```python
from build123d import *

# Parameters (mm, degrees)
SKETCH1_R           = 3.302
BOSS_EXTRUDE1_DEPTH = 19.05
CHAMFER1_SIZE       = 6.593417442
CHAMFER1_SIZE_2     = 6.35
FILLET1_R           = 5.08
FILLET2_R           = 1.27
FILLET3_R           = 1.27
BOSS_EXTRUDE2_START = 38.1
BOSS_EXTRUDE2_DEPTH = 38.1
FILLET5_R           = 2.54
FILLET6_R           = 1.27
SKETCH7_W           = 12.7
SKETCH7_H           = 19.05
BOSS_EXTRUDE3_DEPTH = 12.7
CUT_EXTRUDE5_REACH  = 244.877
SKETCH8_R           = 3.302
SKETCH9_W           = 12.7
SKETCH9_H           = 19.05
BOSS_EXTRUDE4_DEPTH = 12.7
CUT_EXTRUDE6_REACH  = 261.3
SKETCH10_R          = 3.302
FILLET7_R           = 1.27


with BuildPart() as part:
    # Sketch1 → Boss-Extrude1 (new body)
    with BuildSketch(Plane(origin=(0, 0, 0), x_dir=(1, 0, 0), z_dir=(0, 1, 0))):
        with BuildLine():
            Line((0, 0), (0, -107.95))
            ThreePointArc((0, -107.95), (44.047088178, -127.137896363), (63.234984541, -171.184984541))
            Line((63.234984541, -171.184984541), (171.184984541, -171.184984541))
            Line((171.184984541, -171.184984541), (171.184984541, -172.327984541))
            Line((171.184984541, -172.327984541), (173.724984541, -172.327984541))
            Line((173.724984541, -172.327984541), (171.184984541, -168.644984541))
            Line((171.184984541, -168.644984541), (171.184984541, -139.434984541))
            Line((171.184984541, -139.434984541), (158.484984541, -139.434984541))
            Line((158.484984541, -139.434984541), (158.484984541, -152.134984541))
            Line((158.484984541, -152.134984541), (78.172986392, -152.134984541))
            ThreePointArc((78.172986392, -152.134984541), (56.455029962, -114.729954579), (19.05, -93.011998149))
            Line((19.05, -93.011998149), (19.05, -12.7))
            Line((19.05, -12.7), (31.75, -12.7))
            Line((31.75, -12.7), (31.75, 0))
            Line((31.75, 0), (2.54, 0))
            Line((2.54, 0), (-1.143, 2.54))
            Line((-1.143, 2.54), (-1.143, 0))
            Line((-1.143, 0), (0, 0))
        make_face()
        with Locations(Location((25.4, -6.35, 0), (0, 0, 90))):
            Circle(SKETCH1_R, mode=Mode.SUBTRACT)
        with Locations(Location((164.834984541, -145.784984541, 0), (0, 0, 90))):
            Circle(SKETCH1_R, mode=Mode.SUBTRACT)
    extrude(amount=BOSS_EXTRUDE1_DEPTH)

    # Chamfer1
    # the kernel refuses this chamfer: 6.593417442, 6.35 mm, written as the material it takes off along each edge
    with BuildSketch(Plane(origin=(63.234984541, -17.246656522, 171.184984541), x_dir=(-0.0872058515963271, 0, -0.9961903128656489), z_dir=(0, 1, 0))) as chamfer1_piece_1:
        with BuildLine():
            Line((6.700635555, 0), (-CHAMFER1_SIZE * 0.0872058515927, -CHAMFER1_SIZE * 0.996190312824))
            Line((-CHAMFER1_SIZE * 0.0872058515927, -CHAMFER1_SIZE * 0.996190312824), (0, 0))
            ThreePointArc((0, 0), (3.448459053, -0.085459063), (6.700635555, 0))
        make_face()
    extrude(amount=53.543313044, mode=Mode.SUBTRACT)
    with BuildSketch(Plane(origin=(0, -18.02411909, 107.95), x_dir=(0, 0, -1), z_dir=(0, 1, 0))) as chamfer1_piece_2:
        with BuildLine():
            Line((CHAMFER1_SIZE_2, 0), (-0.627104296, -6.977104296))
            ThreePointArc((-0.627104296, -6.977104296), (-0.229600221, -3.597999822), (0, 0))
            Line((0, 0), (CHAMFER1_SIZE_2, 0))
        make_face()
    extrude(amount=55.098238181, mode=Mode.SUBTRACT)

    # Fillet1
    fillet1_edges = [part.edges().sort_by_distance(p)[0] for p in [
        (19.05, 9.525, 93.011998149),
        (78.172986392, 9.525, 152.134984541),
    ]]
    fillet(fillet1_edges, radius=FILLET1_R)

    # Fillet2
    fillet2_edges = [part.edges().sort_by_distance(p)[0] for p in [
        (158.484984541, 19.05, 145.784984541),
        (120.223999201, 19.05, 152.134984541),
        (31.75, 0, 6.35),
        (25.4, 0, 12.7),
        (120.223999201, 0, 152.134984541),
        (158.484984541, 0, 145.784984541),
        (164.834984541, 0, 139.434984541),
        (25.4, 19.05, 12.7),
        (31.75, 9.525, 0),
        (31.75, 9.525, 12.7),
        (158.484984541, 9.525, 139.434984541),
        (171.184984541, 9.525, 139.434984541),
        (31.75, 19.05, 6.35),
        (44.154800127, 19.05, 127.245858784),
        (66.239525947, 19.05, 167.847430426),
        (56.455029962, 0, 114.729954579),
        (56.455029962, 19.05, 114.729954579),
        (19.05, 0, 50.96098534),
        (19.05, 19.05, 50.96098534),
        (78.969227792, 0, 151.159085536),
        (78.969227792, 19.05, 151.159085536),
        (20.025899005, 0, 92.215756749),
        (20.025899005, 19.05, 92.215756749),
        (164.834984541, 19.05, 139.434984541),
    ]]
    fillet(fillet2_edges, radius=FILLET2_R)

    # Fillet3
    fillet3_edges = [part.edges().sort_by_distance(p)[0] for p in [
        (120.506693262, 0, 171.184984541),
    ]]
    fillet(fillet3_edges, radius=FILLET3_R)

    # Sketch6 → Boss-Extrude2 (add)
    with BuildSketch(Plane.XZ.offset(BOSS_EXTRUDE2_START)):
        with BuildLine():
            Line((6.977104296, 108.577104296), (14.376413508, 105.755665739))
            ThreePointArc((14.376413508, 105.755665739), (47.125159878, 124.289265483), (65.50643038, 157.123753494))
            Line((65.50643038, 157.123753494), (62.650649911, 164.509876311))
            ThreePointArc((62.650649911, 164.509876311), (44.154800127, 127.245858784), (6.977104296, 108.577104296))
        make_face()
    extrude(amount=-BOSS_EXTRUDE2_DEPTH)

    # Fillet5
    # the kernel refuses this fillet: 2.54 mm, written as the material it takes off along each edge
    with BuildSketch(Plane(origin=(173.724984541, -9.855086022, 172.327984541), x_dir=(-0.5677329558036762, 0, -0.8232127859152948), z_dir=(0, 1, 0))) as fillet5_piece_1:
        with BuildLine():
            CenterArc((3.942034409, 2.54), FILLET5_R, 190.182679729, 79.817320271)
            Line((1.442041708, 2.090960476), (0, 0))
            Line((0, 0), (3.942034409, 0))
        make_face()
    extrude(amount=38.760172045, mode=Mode.SUBTRACT)
    with BuildSketch(Plane(origin=(-1.143, -9.855086022, -2.54), x_dir=(0, 0, 1), z_dir=(0, 1, 0))) as fillet5_piece_2:
        with BuildLine():
            CenterArc((4.328983323, 1.80309142), FILLET5_R, 145.407711312, 79.817320271)
            Line((2.238022847, 3.245133128), (0, 0))
            Line((0, 0), (2.54, 0))
        make_face()
    extrude(amount=38.760172045, mode=Mode.SUBTRACT)

    # Fillet6
    fillet6_edges = [part.edges().sort_by_distance(p)[0] for p in [
        (47.125159878, -38.1, 124.289265483),
        (64.078540146, -38.1, 160.816814902),
        (44.154800127, -38.1, 127.245858784),
        (10.676758902, -38.1, 107.166385018),
    ]]
    fillet(fillet6_edges, radius=FILLET6_R)

    # Sketch7 → Boss-Extrude3 (add)
    with BuildSketch(Plane(origin=(0, 0, 0), x_dir=(-1, 0, 0), z_dir=(0, 0, -1))):
        with Locations((-11.43, 9.525)):
            Rectangle(SKETCH7_W, SKETCH7_H)
    extrude(amount=BOSS_EXTRUDE3_DEPTH)

    # Sketch8 → Cut-Extrude5 (cut, up to next)
    with BuildSketch(Plane.ZY.offset(-5.08), mode=Mode.PRIVATE) as cut_extrude5_sk1:
        with Locations((-6.35, 9.525)):
            Circle(SKETCH8_R)
    cut_extrude5_tool1 = extrude(cut_extrude5_sk1.sketch, amount=-CUT_EXTRUDE5_REACH, mode=Mode.PRIVATE) & part.part
    add(cut_extrude5_tool1.solids().sort_by_distance((5.08, 9.525, -6.35))[0], mode=Mode.SUBTRACT)

    # Sketch9 → Boss-Extrude4 (add)
    with BuildSketch(Plane(origin=(171.184984541, 0, -171.184984541), x_dir=(0, 0, 1), z_dir=(-1, 0, 0))):
        with Locations((330.939969082, 9.525)):
            Rectangle(SKETCH9_W, SKETCH9_H)
    extrude(amount=-BOSS_EXTRUDE4_DEPTH)

    # Sketch10 → Cut-Extrude6 (cut, up to next)
    with BuildSketch(Plane.XY.offset(166.104984541), mode=Mode.PRIVATE) as cut_extrude6_sk1:
        with Locations((177.534984541, 9.525)):
            Circle(SKETCH10_R)
    cut_extrude6_tool1 = extrude(cut_extrude6_sk1.sketch, amount=-CUT_EXTRUDE6_REACH, mode=Mode.PRIVATE) & part.part
    add(cut_extrude6_tool1.solids().sort_by_distance((177.534985, 9.525, 166.104985))[0], mode=Mode.SUBTRACT)

    # Fillet7
    fillet7_edges = [part.edges().sort_by_distance(p)[0] for p in [
        (17.78, 9.525, -12.7),
        (11.43, 0, -12.7),
        (5.08, 9.525, -12.7),
        (11.43, 19.05, -12.7),
        (183.884984541, 9.525, 153.404984541),
        (183.884984541, 19.05, 159.754984541),
        (183.884984541, 9.525, 166.104984541),
        (183.884984541, 0, 159.754984541),
    ]]
    fillet(fillet7_edges, radius=FILLET7_R)


solid = part.part
```
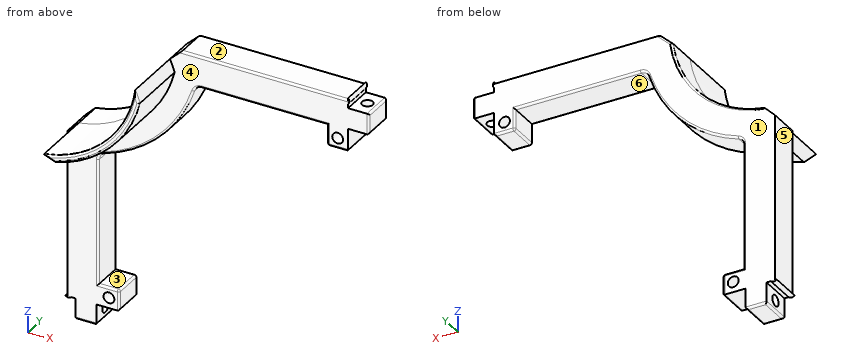
The listing builds one solid part. Answer for the finished solid, in the listing's coordinates (mm). Face numbers are marked on the shaded views. A direction names the side the tool comes from. Give positions to 0.01 mm unless a question says otherwise; leave off trailing zeros. Loops run counter-clockwise (first coordinate to the right, second up) from the corner with the lowest first, then second, coordinate; pieces in that order, holes last. Notation, with made-up numbers: M 81,24 L 112,24 A29 ccw 112,44 Z; hole C 67,7.5 d8. An arc over 180 degrees is marked long. One line per item, written item: value.
Q1. For the marked faces 1, 2 and 3, determine the directions among +Z, -Z, +X, -X, +Y, -Y from which every point of the face is accessible in a straight line to the end or side of a thin tool.
Working result:
face 1: +Z, -Z, +X, -X, +Y
face 2: +Z, -X, +Y, -Y
face 3: +X, +Y, -Y
Q2. A cutting plane is placed at C-C on y = -16.5. Determine the outline of the cut face in (x, z), then the cut area to 3 significant figures.
Working result:
outline: M 6.98,108.58 L 14.38,105.76 A69.85 ccw 65.51,157.12 L 62.65,164.51 A65.66 cw Z
area: 336 mm^2
Q3. Determine the mould class of the marked faces 4, 5 and 6 for opening direction X: +X half, -X half, draft (parallel to the pull), parting line (faces both ways), or undercut.
Working result:
face 4: draft
face 5: -X half
face 6: undercut
Q4. Find the intervals of material crossed by line 1 (Z direction, x = 25.4, y = 6.25); line 2 (Y direction, x = 14, z = -6); line 3 (Z direction, x = 25, y = 7), in increasing order. Write a range as from..to.
Working result:
line 1: z = 0..3.05, 9.65..12.7, 95.02..114.07
line 2: y = 0..6.24, 12.81..19.05
line 3: z = 0..3.07, 9.63..12.7, 94.88..113.89
Q5. A cutting plane is placed at B-B on x = 118.5. Determine the outline of the cut face in (y, z).
Working result:
outline: M 0,153.4 A1.27 ccw 1.27,152.13 L 17.78,152.13 A1.27 ccw 19.05,153.4 L 19.05,171.18 L 1.27,171.18 A1.27 ccw 0,169.91 Z
Q6. A cutting plane is placed at D-D on z = 80. Determine the outline of the cut face in (x, y), then the cut area to 3 significant figures.
Working result:
outline: M 0,0 L 17.78,0 A1.27 ccw 19.05,1.27 L 19.05,17.78 A1.27 ccw 17.78,19.05 L 0,19.05 Z
area: 362 mm^2
Q7. Flat-ended cylindrical pins translate along their axes: P1, Ø0.7, axis at y = 7.5, z = 171, coming from the -X side; P2, Ø3.5, axis at y = 13.5, z = -4.5, coming from the +X side; P3, Ø0.8, axis at x = 3.5, y = 5, coming from the -Z side; P4, Ø12, axis at x = 72.5, y = -7, coming from the -Z side. Find the tip coordinate at first contact, or state that the pin passes through.
Working result:
P1: stops at x = 69.25
P2: stops at x = 17.78
P3: stops at z = 0
P4: passes through
Q8. A cutting plane is placed at A-A on z = -6.35. Determine the outline of the cut face in (x, y), then the cut area to 3 significant figures.
Working result:
outline: M 5.08,0 L 17.78,0 L 17.78,6.22 L 5.08,6.22 Z; M 5.08,12.83 L 17.78,12.83 L 17.78,19.05 L 5.08,19.05 Z
area: 158 mm^2
